Here's how the part is built. I have some questions about the finished solid (model axes, mm). Give positions to 0.01 mm unless a question says otherwise; leave off trailing zeros. Order: outer loops, then holes, each group sorted by start corner. A loop starts at its lowest first (then second) coordinate and runs counter-clockwise, first axis right, second up.
from build123d import *

# Parameters (mm, degrees)
SKETCH_1_R      = 29.29
EXTRUDE_1_DEPTH = 0.5


with BuildPart() as part:
    # 草图1 → 凸台-拉伸1 (new body)
    with BuildSketch(Plane(origin=(0, 0, 0), x_dir=(1, 0, 0), z_dir=(0, 1, 0))):
        with BuildLine():
            Line((-10, -92.088636107), (-10, -112.088636107))
            Line((-10, -112.088636107), (10, -112.088636107))
            Line((10, -112.088636107), (10, -92.088636107))
            ThreePointArc((10, -92.088636107), (0, 92.63), (-10, -92.088636107))
        make_face()
        with Locations(Location((0, 0, 0), (0, 0, 270))):
            Circle(SKETCH_1_R, mode=Mode.SUBTRACT)
        with BuildLine():
            Line((-2, -41.37168597), (-2, -50.690560265))
            ThreePointArc((-2, -50.690560265), (-43.933468734, -25.365), (-44.899312922, 23.613229325))
            Line((-44.899312922, 23.613229325), (-36.828931047, 18.953792177))
            ThreePointArc((-36.828931047, 18.953792177), (-35.870772225, -20.71), (-2, -41.37168597))
        make_face(mode=Mode.SUBTRACT)
        with BuildLine():
            Line((2, -41.37168597), (2, -50.690560265))
            ThreePointArc((2, -50.690560265), (43.933468734, -25.365), (44.899312922, 23.613229325))
            Line((44.899312922, 23.613229325), (36.828931047, 18.953792177))
            ThreePointArc((36.828931047, 18.953792177), (35.870772225, -20.71), (2, -41.37168597))
        make_face(mode=Mode.SUBTRACT)
        with BuildLine():
            Line((-34.828931047, 22.417893793), (-42.899312922, 27.07733094))
            ThreePointArc((-42.899312922, 27.07733094), (0, 50.73), (42.899312922, 27.07733094))
            Line((42.899312922, 27.07733094), (34.828931047, 22.417893793))
            ThreePointArc((34.828931047, 22.417893793), (0, 41.42), (-34.828931047, 22.417893793))
        make_face(mode=Mode.SUBTRACT)
        with BuildLine():
            Line((51.70219226, 27.540873542), (57.698214258, 31.002678457))
            ThreePointArc((57.698214258, 31.002678457), (56.724663948, -32.75), (2, -65.469458528))
            Line((2, -65.469458528), (2, -58.5458487))
            ThreePointArc((2, -58.5458487), (50.731768154, -29.29), (51.70219226, 27.540873542))
        make_face(mode=Mode.SUBTRACT)
        with BuildLine():
            Line((49.70219226, 31.004975158), (55.698214258, 34.466780072))
            ThreePointArc((55.698214258, 34.466780072), (0, 65.5), (-55.698214258, 34.466780072))
            Line((-55.698214258, 34.466780072), (-49.70219226, 31.004975158))
            ThreePointArc((-49.70219226, 31.004975158), (0, 58.58), (49.70219226, 31.004975158))
        make_face(mode=Mode.SUBTRACT)
        with BuildLine():
            Line((63.11317795, 34.129009202), (68.094616028, 37.005043818))
            ThreePointArc((68.094616028, 37.005043818), (67.116968793, -38.75), (2, -77.47418925))
            Line((2, -77.47418925), (2, -71.722120019))
            ThreePointArc((2, -71.722120019), (62.137322722, -35.875), (63.11317795, 34.129009202))
        make_face(mode=Mode.SUBTRACT)
        with BuildLine():
            Line((61.11317795, 37.593110817), (66.094616028, 40.469145433))
            ThreePointArc((66.094616028, 40.469145433), (0, 77.5), (-66.094616028, 40.469145433))
            Line((-66.094616028, 40.469145433), (-61.11317795, 37.593110817))
            ThreePointArc((-61.11317795, 37.593110817), (0, 71.75), (61.11317795, 37.593110817))
        make_face(mode=Mode.SUBTRACT)
        with BuildLine():
            Line((72.729295793, 39.680877427), (77.077938162, 42.19156727))
            ThreePointArc((77.077938162, 42.19156727), (76.097652231, -43.935), (2, -87.847236155))
            Line((2, -87.847236155), (2, -82.82585647))
            ThreePointArc((2, -82.82585647), (71.750204704, -41.425), (72.729295793, 39.680877427))
        make_face(mode=Mode.SUBTRACT)
        with BuildLine():
            Line((70.729295793, 43.144979043), (75.077938162, 45.655668885))
            ThreePointArc((75.077938162, 45.655668885), (0, 87.87), (-75.077938162, 45.655668885))
            Line((-75.077938162, 45.655668885), (-70.729295793, 43.144979043))
            ThreePointArc((-70.729295793, 43.144979043), (0, 82.85), (70.729295793, 43.144979043))
        make_face(mode=Mode.SUBTRACT)
        with BuildLine():
            Line((-51.70219226, 27.540873542), (-57.698214258, 31.002678457))
            ThreePointArc((-57.698214258, 31.002678457), (-56.724663948, -32.75), (-2, -65.469458528))
            Line((-2, -65.469458528), (-2, -58.5458487))
            ThreePointArc((-2, -58.5458487), (-50.731768154, -29.29), (-51.70219226, 27.540873542))
        make_face(mode=Mode.SUBTRACT)
        with BuildLine():
            Line((-63.11317795, 34.129009202), (-68.094616028, 37.005043818))
            ThreePointArc((-68.094616028, 37.005043818), (-67.116968793, -38.75), (-2, -77.47418925))
            Line((-2, -77.47418925), (-2, -71.722120019))
            ThreePointArc((-2, -71.722120019), (-62.137322722, -35.875), (-63.11317795, 34.129009202))
        make_face(mode=Mode.SUBTRACT)
        with BuildLine():
            Line((-72.729295793, 39.680877427), (-77.077938162, 42.19156727))
            ThreePointArc((-77.077938162, 42.19156727), (-76.097652231, -43.935), (-2, -87.847236155))
            Line((-2, -87.847236155), (-2, -82.82585647))
            ThreePointArc((-2, -82.82585647), (-71.750204704, -41.425), (-72.729295793, 39.680877427))
        make_face(mode=Mode.SUBTRACT)
    extrude(amount=EXTRUDE_1_DEPTH)


solid = part.part
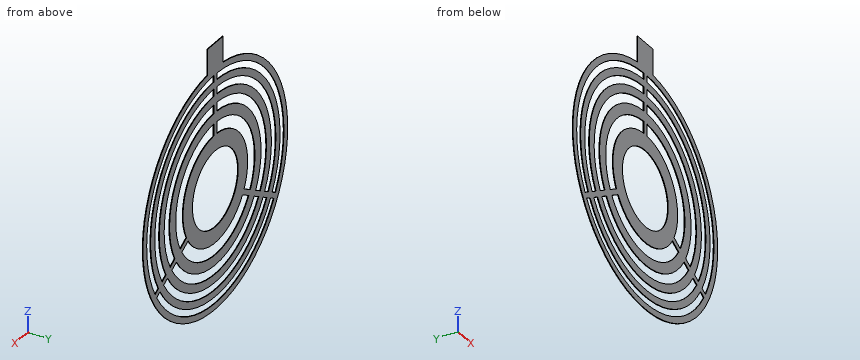
Q1. If we section it at C-C on z = 0: Give the number of separate pieces and of enclosed holes in the cut face, plus the area to 3 significant figures.
Filled sheet:
separate pieces: 10
enclosed holes: 0
area: 36.3 mm2
Q2. If we section it at B-B on z = 53.5: List the corners of the cut face in (x, y) for me.
Filled sheet:
outline: (-75.62, 0) - (-69.71, 0) - (-69.71, 0.5) - (-75.62, 0.5) - close; (-63.26, 0) - (-56.07, 0) - (-56.07, 0.5) - (-63.26, 0.5) - close; (-47.81, 0) - (-37.79, 0) - (-37.79, 0.5) - (-47.81, 0.5) - close; (-23.86, 0) - (23.86, 0) - (23.86, 0.5) - (-23.86, 0.5) - close; (37.79, 0) - (47.81, 0) - (47.81, 0.5) - (37.79, 0.5) - close; (56.07, 0) - (63.26, 0) - (63.26, 0.5) - (56.07, 0.5) - close; (69.71, 0) - (75.62, 0) - (75.62, 0.5) - (69.71, 0.5) - close
Q3. If we section it at A-A on z = 80: List the corners of the cut face in (x, y) for me, plus the area to 3 significant figures.
Filled sheet:
outline: (-46.69, 0) - (-36.35, 0) - (-36.35, 0.5) - (-46.69, 0.5) - close; (-21.54, 0) - (21.54, 0) - (21.54, 0.5) - (-21.54, 0.5) - close; (36.35, 0) - (46.69, 0) - (46.69, 0.5) - (36.35, 0.5) - close
area: 31.9 mm2
Q4. I need wall thicknesses on L1, parallel to Z at x = -59.5, y = 0.4. Which ranges of the line are inside material? Lowest first, please.
Filled sheet:
L1: z = -70.99 to -64.66, -57.65 to -49.66, -40.1 to -27.39, 27.39 to 40.1, 49.66 to 57.65, 64.66 to 70.99
